Model file for the job. Use its own axes, mm. A direction names the side the tool comes from. Round coordinates to 2 decimals unless told otherwise and drop trailing zeros. Loops run counter-clockwise (first coordinate to the right, second up) from the corner with the lowest first, then second, coordinate; pieces in that order, holes last. Notation, with made-up numbers: M -13.75,39.25 L 5.25,39.25 A18 ccw 5.25,71.25 Z; hole C -28.5,-2 d9. An arc over 180 degrees is marked long. Use a Markdown table: item, result. Add a question column.
Item 1: Two-plate mould, pull along Z, no slides. Class faces 1 (the cylindrical face through (-60.257, -3.863, 77.68)), 2 (the flat face through (-24, -4, 20.29)), 3 (the flat face through (6.339, -4, 62)): +Z half, -Z half, draft (parallel to the pull), parting line (faces both ways), or undercut.
Item 2: Saw through at B-B on y = -1.25. Write the cut outline in (x, z).
Item 3: Tool access for faces 4 (the flat face through (8, -4, 46.9)), 5 (the cylindrical face through (12.928, -3.863, 26.085)): list every direction of +Z, -Z, +X, -X, +Y, -Y with a clear straight run to the whole face (end or side of a thin tool).
Item 4: Pin check, flat tips, straight feed: P1, Ø1.1, axis at x = 7.5, y = -4.5, coming from the +Z side; P2, Ø4, axis at x = -17.5, z = 64, coming from the +Y side (3 decimals); P3, Ø1, axis at x = 8, y = -4.5, coming from the -Z side; P4, Ø4, axis at x = 9, y = -3, coming from the -Z side. Stop position of each tip, or through.
Item 5: Saw through at C-C on x = -25. Write the cut outline in (y, z).
Item 6: Wall check: L1, parallel to X at y = -7, z = 40.5; L2, parallel to Z at x = -14, y = -2.5; L3, parallel to Z at x = -20.5, y = -6.5. Give the ranges that are in metal, low to high. Write a range as from..to.
Item 7: Saw through at D-D on z = 38.5. Write the cut outline in (x, y), then the cut area to 3 significant figures.
Item 8: Saw through at A-A on x = -51.5. Write the cut outline in (y, z).
```python
from build123d import *

# Parameters (mm, degrees)
F0_W     = 85.09
F0_H     = 63.5
F0_R     = 3.81
F1_DEPTH = 7.62
F2_R     = 20.32


with BuildPart() as f1:
    # F0 (on Front) → F1 (new body)
    with BuildSketch(Plane.XZ):
        with Locations((-23.506424, 52.040306)):
            Rectangle(F0_W, F0_H)
        with Locations((-23.506424, 28.545306)):
            Circle(F0_R, mode=Mode.SUBTRACT)
        Polygon((-53.364091, 67.207848), (-42.140279, 67.207848), (6.338576, 67.207848), (6.338576, 57.047848), (10.148576, 57.047848), (10.206486, 46.900329), (6.396486, 46.900329), (6.396486, 36.740329), (-53.364091, 36.727848), align=None, mode=Mode.SUBTRACT)
        with Locations((-23.506424, 75.535306)):
            Circle(F0_R, mode=Mode.SUBTRACT)
    extrude(amount=F1_DEPTH)

    # F2
    f2_edges = [f1.edges().sort_by_distance(p)[0] for p in [
        (-66.051424, -3.81, 83.790306),
        (-66.051424, -3.81, 20.290306),
        (19.038576, -3.81, 20.290306),
        (19.038576, -3.81, 83.790306),
    ]]
    fillet(f2_edges, radius=F2_R)


solid = f1.part
```
Entries:
| question | item | result |
|---|---|---|
| 1 | face 1 | +Z half |
| 1 | face 2 | -Z half |
| 1 | face 3 | undercut |
| 2 | outline | M -66.05,40.61 A20.32 ccw -45.73,20.29 L -1.28,20.29 A20.32 ccw 19.04,40.61 L 19.04,63.47 A20.32 ccw -1.28,83.79 L -45.73,83.79 A20.32 ccw -66.05,63.47 Z; hole M -53.36,36.73 L 6.4,36.74 L 6.4,46.9 L 10.21,46.9 L 10.15,57.05 L 6.34,57.05 L 6.34,67.21 L -53.36,67.21 Z; hole C -23.51,28.55 d7.62; hole C -23.51,75.54 d7.62 |
| 3 | face 4 | +Y, -Y |
| 3 | face 5 | -Z, +X, +Y, -Y |
| 4 | P1 | z = 82.05 |
| 4 | P2 | through |
| 4 | P3 | z = 22.29 |
| 4 | P4 | z = 22.05 |
| 5 | outline | M -7.62,20.29 L 0,20.29 L 0,25.04 L -7.62,25.04 Z; M -7.62,32.05 L 0,32.05 L 0,36.73 L -7.62,36.73 Z; M -7.62,67.21 L 0,67.21 L 0,72.03 L -7.62,72.03 Z; M -7.62,79.04 L 0,79.04 L 0,83.79 L -7.62,83.79 Z |
| 6 | L1 | -66.05..-53.36, 6.4..19.04 |
| 6 | L2 | 20.29..36.74, 67.21..83.79 |
| 6 | L3 | 20.29..26.2, 30.89..36.73, 67.21..73.19, 77.88..83.79 |
| 7 | outline | M -65.94,-7.62 L -53.36,-7.62 L -53.36,0 L -65.94,0 Z; M 6.4,-7.62 L 18.93,-7.62 L 18.93,0 L 6.4,0 Z |
| 7 | area | 191 mm2 |
| 8 | outline | M -7.62,21.13 L 0,21.13 L 0,36.73 L -7.62,36.73 Z; M -7.62,67.21 L 0,67.21 L 0,82.95 L -7.62,82.95 Z |
